For this review, take the finished solid that the model builds, in its own axes (mm). Face numbers are marked on the shaded views. A direction names the side the tool comes from. Round coordinates to 2 decimals unless told otherwise and drop trailing zeros. Write each loop counter-clockwise with the first axis right and the second up, starting at its lowest first coordinate (ties: lowest second). Pieces come first, ordered by that corner, then holes. Notation, with made-up numbers: M 74.25,41.5 L 120.25,41.5 A20 ccw 120.25,72.5 Z; hole C 0.5,-26.5 d4. An arc over 180 degrees is marked long. Write each question's results on one line, items separated by ' | '. Start each with the question number.
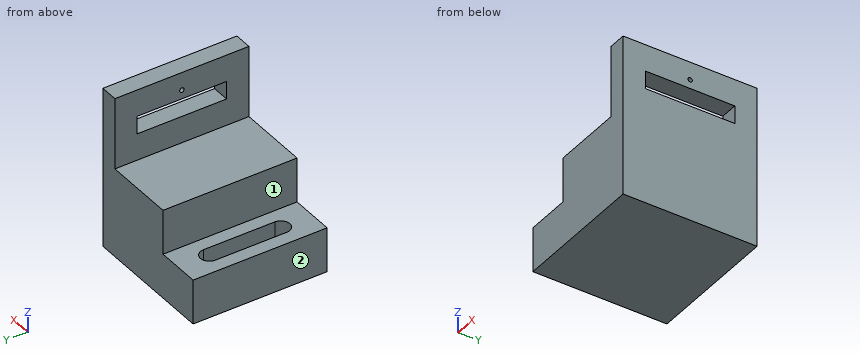
```python
from build123d import *

# Parameters (mm, degrees)
F1_DEPTH = 150
F2_W     = 100
F2_H     = 20
F3_DEPTH = 20.001
F6_DEPTH = 25
F4_R     = 2.5
F7_DEPTH = 20.001


with BuildPart() as f1:
    # F0 (on Front) → F1 (new body)
    with BuildSketch(Plane.XZ):
        Polygon((75, -90), (75, 90), (55, 90), (55, 10), (-25, 10), (-25, -40), (-75, -40), (-75, -90), align=None)
    extrude(amount=F1_DEPTH)

    # F2 (on face) → F3 (cut, through all)
    with BuildSketch(Plane(origin=(55, 0, 0), x_dir=(0, -1, 0), z_dir=(-1, 0, 0))):
        with Locations((75, 50)):
            Rectangle(F2_W, F2_H)
    extrude(amount=-F3_DEPTH, mode=Mode.SUBTRACT)

    # F5 (on face) → F6 (cut)
    with BuildSketch(Plane.XY.offset(-40)):
        with BuildLine():
            ThreePointArc((-40, -35), (-50, -25), (-60, -35))
            Line((-60, -35), (-60, -115))
            ThreePointArc((-60, -115), (-50, -125), (-40, -115))
            Line((-40, -115), (-40, -35))
        make_face()
    extrude(amount=-F6_DEPTH, mode=Mode.SUBTRACT)

    # F4 (on face) → F7 (cut, through all)
    with BuildSketch(Plane(origin=(55, 0, 0), x_dir=(0, -1, 0), z_dir=(-1, 0, 0))):
        with Locations((75, 70)):
            Circle(F4_R)
    extrude(amount=-F7_DEPTH, mode=Mode.SUBTRACT)


solid = f1.part
```
Item 1: We need section D-D on z = -50. State the section outline as (x, y) points, then the cut area to 3 significant figures.
Item 2: We need section C-C on x = 63. State the section outline as (y, z) points.
Item 3: Insertion check: P1, Ø1.5, axis at y = -68.5, z = -23, coming from the -X side; P2, Ø4, axis at x = 8, y = -67, coming from the +Z side; P3, Ø10, axis at x = -54.5, y = -75.5, coming from the +Z side; P4, Ø5, axis at x = -43, z = -55.5, coming from the +Y side. Each pin has a flat end and moves straight along its axis. Give the tip position at first contact, or say it passes through.
Item 4: We need section B-B on z = 70. State the section outline as (x, y) points.
Item 5: For the marked faces 1 and 2, list the 3-axis set-ups (+Z, -Z, +X, -X, +Y, -Y) from which the entire face can be reached by the end or side of a thin tool; tool diameter is ignored.
Item 6: For probe 1 along Z at (x, y) = (67.75, -75); probe 2 along Z at (x, y) = (65, -82); probe 3 along Z at (x, y) = (-26, -103.5), list the stretches that pass through material, from the lowest coordinate up.
Item 7: We need section A-A on y = -121. State the section outline as (x, z) points.
Numbers:
1) outline: M -75,-150 L 75,-150 L 75,0 L -75,0 Z; hole M -60,-115 A10 ccw -40,-115 L -40,-35 A10 ccw -60,-35 Z | area: 20,600 mm^2
2) outline: M -150,-90 L 0,-90 L 0,90 L -150,90 Z; hole M -125,40 L -25,40 L -25,60 L -125,60 Z; hole C -75,70 d5
3) P1: stops at x = -25 | P2: stops at z = 10 | P3: stops at z = -65 | P4: stops at y = 0
4) outline: M 55,-150 L 75,-150 L 75,-77.5 L 55,-77.5 Z; M 55,-72.5 L 75,-72.5 L 75,0 L 55,0 Z
5) face 1: +Z, -X, +Y, -Y | face 2: +Z, -Z, -X, +Y, -Y
6) probe 1: z = -90 to 40, 60 to 67.5, 72.5 to 90 | probe 2: z = -90 to 40, 60 to 90 | probe 3: z = -90 to -40
7) outline: M -75,-90 L 75,-90 L 75,40 L 55,40 L 55,10 L -25,10 L -25,-40 L -42,-40 L -42,-65 L -58,-65 L -58,-40 L -75,-40 Z; M 55,60 L 75,60 L 75,90 L 55,90 Z
